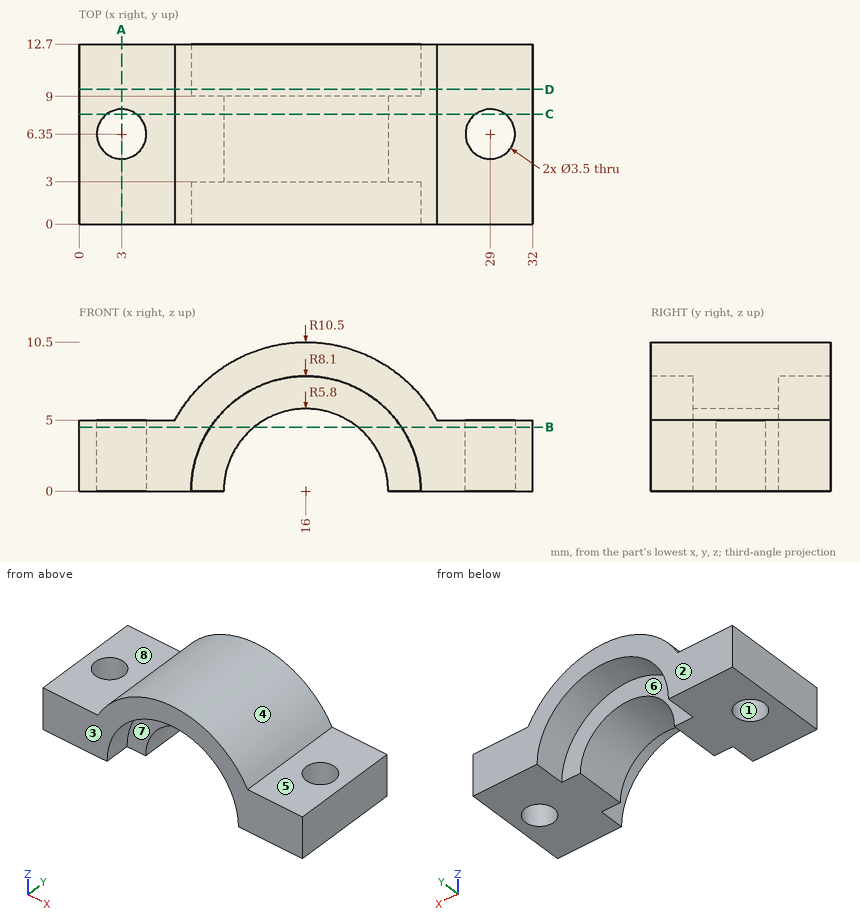
Could you check a few things on this drawing? It's one solid part, dimensions in mm from its lowest x, y, z. A direction names the side the tool comes from. Round coordinates to 2 decimals unless told otherwise and drop trailing zeros. Write each loop counter-clockwise with the first axis right and the second up, starting at its lowest first coordinate (ties: lowest second). Pieces come first, ordered by that corner, then holes. Notation, with made-up numbers: (-31.5, 71.5) -> (-16.5, 71.5) arc R14 ccw to (-16.5, 95.5) -> close; hole circle Ø5 at (52.25, -22). An arc over 180 degrees is marked (long way). One line per item, written item: value.
1) We'd pull the mould along Y, two halves only. Please class the marked faces 1, 2, 3 and 4: released by +Y, released by -Y, zero draft, split by the parting line, or undercut.
Filled sheet:
face 1: undercut
face 2: released by +Y
face 3: released by -Y
face 4: zero draft
2) If I drill on line 1 (Y direction, x = 3, z = 3.2); line 2 (X direction, y = 7, z = 3); line 3 (Y direction, x = 16, z = 6), over which ranges is the centre line in solid material (lowest first)? Write a range as [from, to].
Filled sheet:
line 1: y = [0, 4.6], [8.1, 12.7]
line 2: x = [0, 1.38], [4.62, 11.04], [20.96, 27.38], [30.62, 32]
line 3: y = [3, 9]
3) For the marked faces 5, 6, 7 and 8, which set-ups out of +Z, -Z, +X, -X, +Y, -Y let a thin tool reach every point of the face, with its end or its side?
Filled sheet:
face 5: +Z, +X, +Y, -Y
face 6: -Z, +Y
face 7: -Z, -Y
face 8: +Z, -X, +Y, -Y
4) Suppose I cut it at B-B on z = 4.5. List the corners of the cut face in (x, y) for me, plus the area to 3 significant figures.
Filled sheet:
outline: (0, 0) -> (9.27, 0) -> (9.27, 3) -> (12.34, 3) -> (12.34, 9) -> (9.27, 9) -> (9.27, 12.7) -> (0, 12.7) -> close; (19.66, 3) -> (22.73, 3) -> (22.73, 0) -> (32, 0) -> (32, 12.7) -> (22.73, 12.7) -> (22.73, 9) -> (19.66, 9) -> close; hole circle Ø3.5 at (3, 6.35); hole circle Ø3.5 at (29, 6.35)
area: 253 mm2
5) Suppose I cut it at A-A on x = 3. List the corners of the cut face in (y, z) for me, plus the area to 3 significant figures.
Filled sheet:
outline: (0, 0) -> (4.6, 0) -> (4.6, 5) -> (0, 5) -> close; (8.1, 0) -> (12.7, 0) -> (12.7, 5) -> (8.1, 5) -> close
area: 46.0 mm2
6) I'm going to push flat-ended pins straight in: pin 1 Ø5.5 at (x, y) = (29, 6.35) entering from +Z; pin 2 Ø1.5 at (x, z) = (17.5, 5.5) entering from -Y; pin 3 Ø1 at (x, y) = (19, 8.5) entering from +Z; pin 4 Ø6 at (x, z) = (8.5, 2) entering from +Y. Where does each tip first touch, or does it pass through?
Filled sheet:
pin 1: stops at z = 5
pin 2: stops at y = 3
pin 3: stops at z = 10.2
pin 4: stops at y = 12.7
7) Suppose I cut it at D-D on y = 9.5. List the corners of the cut face in (x, z) for me, plus the area to 3 significant figures.
Filled sheet:
outline: (0, 0) -> (7.9, 0) arc R8.1 cw to (24.1, 0) -> (32, 0) -> (32, 5) -> (25.23, 5) arc R10.5 ccw to (6.77, 5) -> (0, 5) -> close
area: 129 mm2
8) Suppose I cut it at C-C on y = 7.75. List the corners of the cut face in (x, z) for me.
Filled sheet:
outline: (0, 0) -> (1.95, 0) -> (1.95, 5) -> (0, 5) -> close; (4.05, 0) -> (10.2, 0) arc R5.8 cw to (21.8, 0) -> (27.95, 0) -> (27.95, 5) -> (25.23, 5) arc R10.5 ccw to (6.77, 5) -> (4.05, 5) -> close; (30.05, 0) -> (32, 0) -> (32, 5) -> (30.05, 5) -> close
